```python
from build123d import *
from OCP.BRepFilletAPI import BRepFilletAPI_MakeChamfer
from build123d.topology import SkipClean

# Parameters (mm, degrees)
ESQUISSE1_R             = 1.5
BOSS_EXTRU_1_DEPTH      = 5
BOSS_EXTRU_3_START      = 8
ESQUISSE3_R             = 1.5
BOSS_EXTRU_3_DEPTH      = 8
ESQUISSE4_W             = 2
ESQUISSE4_H             = 4
ESQUISSE4_H_2           = 3
BOSS_EXTRU_4_DEPTH      = 4
ESQUISSE5_W             = 7
ESQUISSE5_H             = 3
ENL_V_MAT_EXTRU_1_DEPTH = 4
CHANFREIN2_SIZE         = 4.5
CHANFREIN2_SIZE2        = 2.6
CHANFREIN3_SIZE         = 2.6
CHANFREIN3_SIZE2        = 4.5


with BuildPart() as part:
    # Esquisse1 → Boss.-Extru.1 (new body)
    with BuildSketch(Plane.XY):
        Polygon((2.690598923, 4.660254038), (-2.690598923, 4.660254038), (-5.381197846, 0), (-2.690598923, -4.660254038), (2.690598923, -4.660254038), (5.381197846, 0), align=None)
        Circle(ESQUISSE1_R, mode=Mode.SUBTRACT)
    boss_extru_1 = extrude(amount=BOSS_EXTRU_1_DEPTH)

    # Esquisse3 → Boss.-Extru.3 (add)
    with SkipClean():  # the faces are left unmerged after this step: merging them gives an invalid solid
        with BuildSketch(Plane(origin=(0, 0, 0), x_dir=(-1, 0, 0), z_dir=(0, 0, -1)).offset(BOSS_EXTRU_3_START)):
            Polygon((-12, 4.660254038), (10, 4.660254038), (10, -4.660254038), (-12, -4.660254038), (-12, -1.660254038), (-5, -1.660254038), (-5, 0.660254038), (-12, 0.660254038), align=None)
            Circle(ESQUISSE3_R, mode=Mode.SUBTRACT)
        boss_extru_3 = extrude(amount=-BOSS_EXTRU_3_DEPTH)

    # Esquisse4 → Boss.-Extru.4 (add)
    with SkipClean():  # the faces are left unmerged after this step: merging them gives an invalid solid
        with BuildSketch(Plane(origin=(0, 0, -8), x_dir=(-1, 0, 0), z_dir=(0, 0, -1))):
            with Locations((-11, 2.660254038)):
                Rectangle(ESQUISSE4_W, ESQUISSE4_H)
            with Locations((-11, -3.160254038)):
                Rectangle(ESQUISSE4_W, ESQUISSE4_H_2)
        boss_extru_4 = extrude(amount=BOSS_EXTRU_4_DEPTH)

    # Esquisse5 → Enlèv. mat.-Extru.1 (cut)
    with SkipClean():  # the faces are left unmerged after this step: merging them gives an invalid solid
        with BuildSketch(Plane(origin=(0, 4.660254038, 0), x_dir=(1, 0, 0), z_dir=(0, 1, 0))):
            with Locations((8.5, 1.5)):
                Rectangle(ESQUISSE5_W, ESQUISSE5_H)
        enl_v_mat_extru_1 = extrude(amount=-ENL_V_MAT_EXTRU_1_DEPTH, mode=Mode.SUBTRACT)

    # Symétrie3: Boss.-Extru.1, Boss.-Extru.3, Boss.-Extru.4, Enlèv. mat.-Extru.1 across plane
    with SkipClean():  # the faces are left unmerged after this step: merging them gives an invalid solid
        add(boss_extru_1.mirror(Plane.XY.offset(-12)))
        add(boss_extru_3.mirror(Plane.XY.offset(-12)))
        add(boss_extru_4.mirror(Plane.XY.offset(-12)))
        add(enl_v_mat_extru_1.mirror(Plane.XY.offset(-12)), mode=Mode.SUBTRACT)

    # Chanfrein2: one chamfer whose edges measure the first distance from different faces: ONE call of the kernel's chamfer builder (chamfer() names one face for all edges)
    chanfrein2_edges_1 = [part.edges().sort_by_distance(p)[0] for p in [
        (-10, 4.660254038, -4),
    ]]
    chanfrein2_side_1 = [part.faces().sort_by_distance(p)[0] for p in [
        (-10, 0, -4),
    ]]
    chanfrein2_edges_2 = [part.edges().sort_by_distance(p)[0] for p in [
        (-10, -4.660254038, -20),
    ]]
    chanfrein2_side_2 = [part.faces().sort_by_distance(p)[0] for p in [
        (-10, 0, -20),
    ]]
    chanfrein2 = BRepFilletAPI_MakeChamfer(part.part.solid().wrapped)
    for e in chanfrein2_edges_1:
        chanfrein2.Add(CHANFREIN2_SIZE, CHANFREIN2_SIZE2, e.wrapped, chanfrein2_side_1[0].wrapped)  # the first distance lies on this face
    for e in chanfrein2_edges_2:
        chanfrein2.Add(CHANFREIN2_SIZE, CHANFREIN2_SIZE2, e.wrapped, chanfrein2_side_2[0].wrapped)  # the first distance lies on this face
    add(Compound.cast(chanfrein2.Shape()), mode=Mode.REPLACE)

    # Chanfrein3: one chamfer whose edges measure the first distance from different faces: ONE call of the kernel's chamfer builder (chamfer() names one face for all edges)
    chanfrein3_edges_1 = [part.edges().sort_by_distance(p)[0] for p in [
        (-10, -4.660254038, -4),
    ]]
    chanfrein3_side_1 = [part.faces().sort_by_distance(p)[0] for p in [
        (1.3, -4.660254038, -16.404969135),
    ]]
    chanfrein3_edges_2 = [part.edges().sort_by_distance(p)[0] for p in [
        (-10, 4.660254038, -20),
    ]]
    chanfrein3_side_2 = [part.faces().sort_by_distance(p)[0] for p in [
        (-5.045299462, 4.660254038, -0.404969135),
    ]]
    chanfrein3 = BRepFilletAPI_MakeChamfer(part.part.solid().wrapped)
    for e in chanfrein3_edges_1:
        chanfrein3.Add(CHANFREIN3_SIZE, CHANFREIN3_SIZE2, e.wrapped, chanfrein3_side_1[0].wrapped)  # the first distance lies on this face
    for e in chanfrein3_edges_2:
        chanfrein3.Add(CHANFREIN3_SIZE, CHANFREIN3_SIZE2, e.wrapped, chanfrein3_side_2[0].wrapped)  # the first distance lies on this face
    add(Compound.cast(chanfrein3.Shape()), mode=Mode.REPLACE)


solid = part.part
```
Geometry check sheet. Reference: the model listing, model coordinates, mm. A direction names the side the tool comes from. Coordinates: 2 decimals unless noted, no trailing zeros. Write each loop counter-clockwise with the first axis right and the second up, starting at its lowest first coordinate (ties: lowest second). Pieces come first, ordered by that corner, then holes. Notation, with made-up numbers: M 2,42.5 L 21,42.5 A19 cw 21,64.5 Z; hole C 86.5,-0.5 d10. An arc over 180 degrees is marked long. Answer as a JSON object with one key per item and string values.
1. Draft check along Z on faces 1 (the flat face through (5, 0, -21)), 2 (the flat face through (-6, 0, -24)), 3 (the flat face through (-8.718, -2.379, -4.056)), 4 (the flat face through (2, 0, -8)). Enter one of: released by +Z, released by -Z, zero draft, split by the parting line, or undercut.
Answers below:
{"face 1": "undercut", "face 2": "released by -Z", "face 3": "zero draft", "face 4": "undercut"}
2. Scan lines: L1, parallel to Z at x = -2.5, y = -3.75; L2, parallel to Y at x = 0, z = -25.35; L3, parallel to Z at x = 7.75, y = 2.75. Record each from-to range of solid material in increasing order.
Answers below:
{"L1": "z = -29 to -16, -8 to 5", "L2": "y = -4.66 to -1.5, 1.5 to 4.66", "L3": "z = -21 to -16, -8 to -3"}
3. Section check C-C, the plane z = -13. Enter the section's corners in (x, y), plus the area to 3 significant figures.
Answers below:
{"outline": "M 10,-4.66 L 12,-4.66 L 12,-1.66 L 10,-1.66 Z; M 10,0.66 L 12,0.66 L 12,4.66 L 10,4.66 Z", "area": "14.0 mm²"}
4. Section check D-D, the plane x = 0. Enter the section's corners in (y, z).
Answers below:
{"outline": "M -4.66,-29 L -1.5,-29 L -1.5,-16 L -4.66,-16 Z; M -4.66,-8 L -1.5,-8 L -1.5,5 L -4.66,5 Z; M 1.5,-29 L 4.66,-29 L 4.66,-16 L 1.5,-16 Z; M 1.5,-8 L 4.66,-8 L 4.66,5 L 1.5,5 Z"}
5. Section check B-B, the plane x = 2.25. Enter the section's corners in (y, z).
Answers below:
{"outline": "M -4.66,-29 L 4.66,-29 L 4.66,-16 L -4.66,-16 Z; M -4.66,-8 L 4.66,-8 L 4.66,5 L -4.66,5 Z"}
6. Section check A-A, the plane z = -22. Enter the section's corners in (x, y), plus the area to 3 significant figures.
Answers below:
{"outline": "M -10,-0.16 L -7.4,-4.66 L 12,-4.66 L 12,-1.66 L 5,-1.66 L 5,4.66 L -7.4,4.66 L -10,0.16 Z; hole C 0,0 d3", "area": "142 mm²"}
7. Tool access check on faces 5 (the flat face through (4, 4, -24)), 6 (the flat face through (-4.055, -2.298, -26.465)), 7 (the flat face through (10, -3, -12)), 8 (the flat face through (-4.02, 2.36, -26.46)), 9 (the flat face through (-4.02, 2.36, 2.46)). Record the directions out of +Z, -Z, +X, -X, +Y, -Y that give a thin tool (end or side, any length) a straight path to the whole face; none if there is none.
Answers below:
{"face 5": "-Z, +X, +Y", "face 6": "-Z, -X, -Y", "face 7": "-X, +Y, -Y", "face 8": "-Z, -X, +Y", "face 9": "+Z, -X, +Y"}
8. Go/stop test with flat-tipped pins: pin 1 Ø1.2 at (x, y) = (8, -2.5) entering from -Z; pin 2 Ø1 at (y, z) = (-3, -2.5) entering from -X; pin 3 Ø1.8 at (x, y) = (0, 0) entering from +Z; pin 4 Ø1 at (y, z) = (0, -21.5) entering from +X. Record where each tip stops, or that it passes through.
Answers below:
{"pin 1": "stops at z = -24", "pin 2": "stops at x = -8.65", "pin 3": "passes through", "pin 4": "stops at x = 5"}
